```python
from build123d import *

# Parameters (mm, degrees)
BASPROSKE_W     = 40
BASPROSKE_H     = 22.5
TOOTHCUT_DEPTH  = 52.112620751
TEETHCUTS_COUNT = 28
TEETHCUTS_ANGLE = 347.142857143
BORSKE_R        = 5
BORE_DEPTH      = 50.0000508
SCALE1_SCALE    = 2


with BuildPart() as part:
    # BasProSke → Base-Revolve (revolve)
    with BuildSketch(Plane(origin=(0, 0, 0), x_dir=(1, 0, 0), z_dir=(0, 1, 0)), mode=Mode.PRIVATE) as base_revolve_sk:
        with Locations((20, 11.25)):
            Rectangle(BASPROSKE_W, BASPROSKE_H)
    revolve(base_revolve_sk.sketch.rotate(Axis((-10, 0, 0), (1, 0, 0)), 180), axis=Axis((-10, 0, 0), (1, 0, 0)))

    # TooCutSke → ToothCut (cut, through all)
    with BuildSketch(Plane(origin=(0, 0, 0), x_dir=(0, 0, -1), z_dir=(1, 0, 0))):
        with BuildLine():
            ThreePointArc((0.70071741, 19.111158288), (0, 19.124), (-0.70071741, 19.111158288))
            ThreePointArc((-0.70071741, 19.111158288), (-1.220048441, 20.845037035), (-2.098754998, 22.427413418))
            ThreePointArc((-2.098754998, 22.427413418), (0, 22.5254), (2.098754998, 22.427413418))
            ThreePointArc((2.098754998, 22.427413418), (1.220048441, 20.845037035), (0.70071741, 19.111158288))
        make_face()
    toothcut = extrude(amount=TOOTHCUT_DEPTH, mode=Mode.SUBTRACT)

    # TeethCuts: ToothCut ×28 about axis
    teethcuts_axis = Axis((-10, 0, 0), (1, 0, 0))
    for i in range(1, TEETHCUTS_COUNT):
        add(toothcut.rotate(teethcuts_axis, i * TEETHCUTS_ANGLE / (TEETHCUTS_COUNT - 1)), mode=Mode.SUBTRACT)

    # BorSke → Bore (cut, symmetric)
    with BuildSketch(Plane(origin=(0, 0, 0), x_dir=(0, 0, -1), z_dir=(1, 0, 0))):
        with Locations(Location((0, 0, 0), (0, 0, 180))):
            Circle(BORSKE_R)
    extrude(amount=BORE_DEPTH, both=True, mode=Mode.SUBTRACT)


with BuildPart() as part_1:
    # Scale1: scaled about (0, 0, 0)
    add(part.part.scale(SCALE1_SCALE))


solid = part_1.part
```
Check sheet for the modelled part. Datum: model origin and axes. Units: mm. A direction names the side the tool comes from. Give positions to 0.01 mm unless a question says otherwise; leave off trailing zeros. Order: outer loops, then holes, each group sorted by start corner. A loop starts at its lowest first (then second) coordinate and runs counter-clockwise, first axis right, second up. Notation, with made-up numbers: (66.5, -24.5) -> (110.5, -24.5) arc R14 cw to (110.5, 0.5) -> close; hole circle Ø1 at (-2, -19). An arc over 180 degrees is marked (long way). Return JSON: item names as keys, results as strings.
1. Material ranges on probe 1 along Y at (x, z) = (35.5, 0); probe 2 along Y at (x, z) = (71, 38.5); probe 3 along Y at (x, z) = (72.5, -40), recorded low to high. Write a range as [from, to].
From the geometry:
{"probe 1": "[-38.25, -10], [10, 38.25]", "probe 2": "[-23.3, -23.08], [-15.88, -10.64], [-7.15, -1.46], [1.46, 7.15], [10.64, 15.88], [23.08, 23.3]", "probe 3": "[-15.9, -11.58], [-7.06, -1.83], [1.83, 7.06], [11.58, 15.9]"}
2. Cross-section at C-C, the plane y = -21. Record the cut outline in (x, z), plus the area to 3 significant figures.
From the geometry:
{"outline": "(0, -37.1) -> (80, -37.1) -> (80, 37.1) -> (0, 37.1) -> close", "area": "5,940 mm^2"}
3. Go/stop test with flat-tipped pins: P1, Ø10, axis at x = 24.5, z = -19.5, coming from the +Y side; P2, Ø1, axis at y = -13.5, z = -10.5, coming from the -X side; P3, Ø1.5, axis at x = 43, z = 2, coming from the +Y side; P4, Ø4, axis at x = 38, y = 28.5, coming from the -Z side. Record where each tip stops, or that it passes through.
From the geometry:
{"P1": "y = 42.6", "P2": "x = 0", "P3": "y = 42.38", "P4": "z = -32.22"}
4. Mould release check, pull along Y, two halves, no side actions. Record for faces 4 (the cylindrical face through (39.44, -40.04, -11.61)), 5 (the cylindrical face through (39.44, -8.53, -37.285)), 6 (the cylindrical face through (39.44, -11.67, -40.12)), 7 (the cylindrical face through (39.44, 31.083, -27.92)): +Y half, -Y half, draft (parallel to the pull), parting line (faces both ways), or undercut.
From the geometry:
{"face 4": "-Y half", "face 5": "undercut", "face 6": "undercut", "face 7": "+Y half"}
5. Cross-section at A-A, the plane z = 0. Record the cut outline in (x, y), plus the area to 3 significant figures.
From the geometry:
{"outline": "(0, -38.25) -> (80, -38.25) -> (80, -10) -> (0, -10) -> close; (0, 10) -> (80, 10) -> (80, 38.25) -> (0, 38.25) -> close", "area": "4,520 mm^2"}
6. Set-up check for faces 1 (the cylindrical face through (39.44, 0.02, 38.248)), 2 (the cylindrical face through (39.44, 38.541, -15.886)), 3 (the cylindrical face through (39.44, -41.71, 2.45)): record each of +Z, -Z, +X, -X, +Y, -Y from which the full face is reachable in a straight line by a thin tool's end or side.
From the geometry:
{"face 1": "+Z, +X, -X", "face 2": "+X, -X", "face 3": "+X, -X, -Y"}
